CAD build for the part. Positions are in the model's coordinates, mm. A direction names the side the tool comes from. Round coordinates to 2 decimals unless told otherwise and drop trailing zeros. Write each loop counter-clockwise with the first axis right and the second up, starting at its lowest first coordinate (ties: lowest second). Pieces come first, ordered by that corner, then holes. Notation, with made-up numbers: (0, -29.5) - (34, -29.5) arc R7 cw to (34, -17.5) - close; hole circle Ø2 at (86.25, -37.5). An arc over 180 degrees is marked (long way). Answer in a Markdown table with one row per item.
```python
from build123d import *

# Parameters (mm, degrees)
F0_R     = 60
F1_DEPTH = 15
F2_R     = 35
F3_DEPTH = 32
F4_R     = 36
F5_DEPTH = 7
F6_R     = 27.5
F7_DEPTH = 22


with BuildPart() as f1:
    # F0 (on Top) → F1 (new body)
    with BuildSketch(Plane.XY):
        Circle(F0_R)
    extrude(amount=-F1_DEPTH)

    # F2 (on face) → F3 (join)
    with BuildSketch(Plane.XY):
        Circle(F2_R)
    extrude(amount=F3_DEPTH)

    # F4 (on face) → F5 (join)
    with BuildSketch(Plane(origin=(0, 0, -15), x_dir=(1, 0, 0), z_dir=(0, 0, -1))):
        Circle(F4_R)
    extrude(amount=F5_DEPTH)

    # F6 (on face) → F7 (cut)
    with BuildSketch(Plane(origin=(0, 0, -22), x_dir=(1, 0, 0), z_dir=(0, 0, -1))):
        Circle(F6_R)
    extrude(amount=-F7_DEPTH, mode=Mode.SUBTRACT)


solid = f1.part
```
Q1. Pull direction Y, two halves, no side cores. Call faces 4 (the cylindrical face through (-5.961, 26.846, -11.154)), 5 (the cylindrical face through (-59.94, 2.64, -7.4)), 6 (the flat face through (-8.2, 26.5, -22)): released by +Y, released by -Y, zero draft, split by the parting line, or undercut.
Computed:
| item | result |
|---|---|
| face 4 | undercut |
| face 5 | split by the parting line |
| face 6 | zero draft |
Q2. 3-axis set-ups, long thin cutter, end or side, ignore diameter. For faces 1 (the cylindrical face through (-4.686, -35.694, -18.451)), 2 (the cylindrical face through (-28, -21, 16)), 3 (the flat face through (0, 0, 32)): which of +Z, -Z, +X, -X, +Y, -Y reach the whole face in a straight line?
Computed:
| item | result |
|---|---|
| face 1 | -Z |
| face 2 | +Z |
| face 3 | +Z, +X, -X, +Y, -Y |
Q3. Drill centre lines: line 1 (Y direction, x = 0, z = -5.5); line 2 (Y direction, x = 0, z = -16.5); line 3 (Z direction, x = 4.5, y = -54.5). Where is each one in solid material? Low to high.
Computed:
| item | result |
|---|---|
| line 1 | y = -60 to -27.5, 27.5 to 60 |
| line 2 | y = -36 to -27.5, 27.5 to 36 |
| line 3 | z = -15 to 0 |
Q4. Saw through at A-A on y = 0. List the corners of the cut face in (x, z), then the cut area to 3 significant figures.
Computed:
| item | result |
|---|---|
| outline | (-60, -15) - (-36, -15) - (-36, -22) - (-27.5, -22) - (-27.5, 0) - (27.5, 0) - (27.5, -22) - (36, -22) - (36, -15) - (60, -15) - (60, 0) - (35, 0) - (35, 32) - (-35, 32) - (-35, 0) - (-60, 0) - close |
| area | 3,330 mm2 |
Q5. Saw through at B-B on z = -6. List the corners of the cut face in (x, y), then the cut area to 3 significant figures.
Computed:
| item | result |
|---|---|
| outline | circle Ø120 at (0, 0); hole circle Ø55 at (0, 0) |
| area | 8,930 mm2 |
Q6. Saw through at D-D on z = 14. List the corners of the cut face in (x, y), then the cut area to 3 significant figures.
Computed:
| item | result |
|---|---|
| outline | circle Ø70 at (0, 0) |
| area | 3,850 mm2 |
Q7. Flat gauge pins, fed straight in: pin 1 (4 mm diameter, centred on x = 0, z = -16.5, fed in from +Y); pin 2 (6 mm diameter, centred on x = 6.5, z = -2.5, fed in from +Y); pin 3 (6 mm diameter, centred on y = 34, z = -13.5, fed in from -X). Where does each tip first touch, or does it go through?
Computed:
| item | result |
|---|---|
| pin 1 | stops at y = 60 |
| pin 2 | stops at y = 59.9 |
| pin 3 | stops at x = -51.37 |
